from build123d import *

# Parameters (mm, degrees)
FILLET1_R          = 1.5
CUT_EXTRUDE1_DEPTH = 0.5


with BuildPart() as part:
    # Sketch1 → Revolve1 (revolve)
    with BuildSketch(Plane.XY, mode=Mode.PRIVATE) as revolve1_sk:
        Polygon((0, 18.4), (2.8, 18.4), (2.8, 16), (1.45, 16), (1.45, 0.2), (1, 0), (0, 0), align=None)
    revolve(revolve1_sk.sketch.rotate(Axis((0, 0, 0), (0, 1, 0)), 90), axis=Axis((0, 0, 0), (0, 1, 0)))

    # Fillet1
    fillet1_edges = [part.edges().sort_by_distance(p)[0] for p in [
        (0, 18.4, 2.8),
    ]]
    fillet(fillet1_edges, radius=FILLET1_R)

    # Sketch2 → Cut-Extrude1 (cut)
    with BuildSketch(Plane(origin=(0, 18.4, 0), x_dir=(1, 0, 0), z_dir=(0, 1, 0))):
        Polygon((1.75, 0.375), (1.75, -0.375), (0.375, -0.375), (0.375, -1.75), (-0.375, -1.75), (-0.375, -0.375), (-1.75, -0.375), (-1.75, 0.375), (-0.375, 0.375), (-0.375, 1.75), (0.375, 1.75), (0.375, 0.375), align=None)
    extrude(amount=-CUT_EXTRUDE1_DEPTH, mode=Mode.SUBTRACT)


solid = part.part
Here's how the part is built. I have some questions about the finished solid (model axes, mm). A direction names the side the tool comes from. Give positions to 0.01 mm unless a question says otherwise; leave off trailing zeros. Loops run counter-clockwise (first coordinate to the right, second up) from the corner with the lowest first, then second, coordinate; pieces in that order, holes last. Notation, with made-up numbers: (56.5, 63) -> (103.5, 63) arc R23 ccw to (103.5, 86) -> close; hole circle Ø7 at (69.25, 82.25). An arc over 180 degrees is marked (long way). One line per item, written item: value.
Q1. Suppose I cut it at A-A on y = 8.25. Please give me the cut outline in (x, z), then the cut area to 3 significant figures.
Answers follow:
outline: circle Ø2.9 at (0, 0)
area: 6.61 mm^2
Q2. On a 3-axis mill with a long thin cutter (end or side, diameter ignored), from which of +Z, -Z, +X, -X, +Y, -Y can I reach the whole of each face in a straight line? I mean faces 4 (the face through (1.2, 16, -1.2)), 5 (the face through (-0.7, 18.4, -0.7)). Say none if no direction works.
Answers follow:
face 4: -Y
face 5: +Z, -Z, +X, -X, +Y
Q3. We'd pull the mould along Z, two halves only. Please class faces 1 (the face through (-0.06, 7.99, 1.45)), 2 (the face through (0.7, 18.4, 0.7)), 3 (the face through (0, 17.9, 0)): pulls with the +Z half, pulls with the -Z half, needs draft (parallel to the pull), parting line crosses it, or undercut.
Answers follow:
face 1: parting line crosses it
face 2: needs draft
face 3: undercut
Q4. If I drill on line 1 along Y through (x, z) = (0.15, 0.3); line 2 along X through (y, z) = (6.25, 0); line 3 along Z through (x, y) = (0.25, 14.5), over which ranges is the centre line in solid material (lowest first)?
Answers follow:
line 1: 0 to 17.9
line 2: -1.45 to 1.45
line 3: -1.43 to 1.43
Q5. I'm going to push flat-ended pins straight in: pin 1 Ø0.6 at (x, y) = (-1, 18) entering from +Z; pin 2 Ø0.5 at (x, y) = (0, 18) entering from +Z; pin 3 Ø1.5 at (y, z) = (10, -0.5) entering from -X. Where does each tip first touch, or does it pass through?
Answers follow:
pin 1: z = 2.4
pin 2: z = 2.54
pin 3: x = -1.45
